Could you check a few things on this drawing? It's one solid part, dimensions in mm from its lowest x, y, z. Round coordinates to 2 decimals unless told otherwise and drop trailing zeros. Loops run counter-clockwise (first coordinate to the right, second up) from the corner with the lowest first, then second, coordinate; pieces in that order, holes last. Notation, with made-up numbers: M 62.25,6.25 L 102.25,6.25 A24 ccw 102.25,36.25 Z; hole C 33,-29 d9. An arc over 180 degrees is marked long. Return JSON: item names as keys, results as strings.
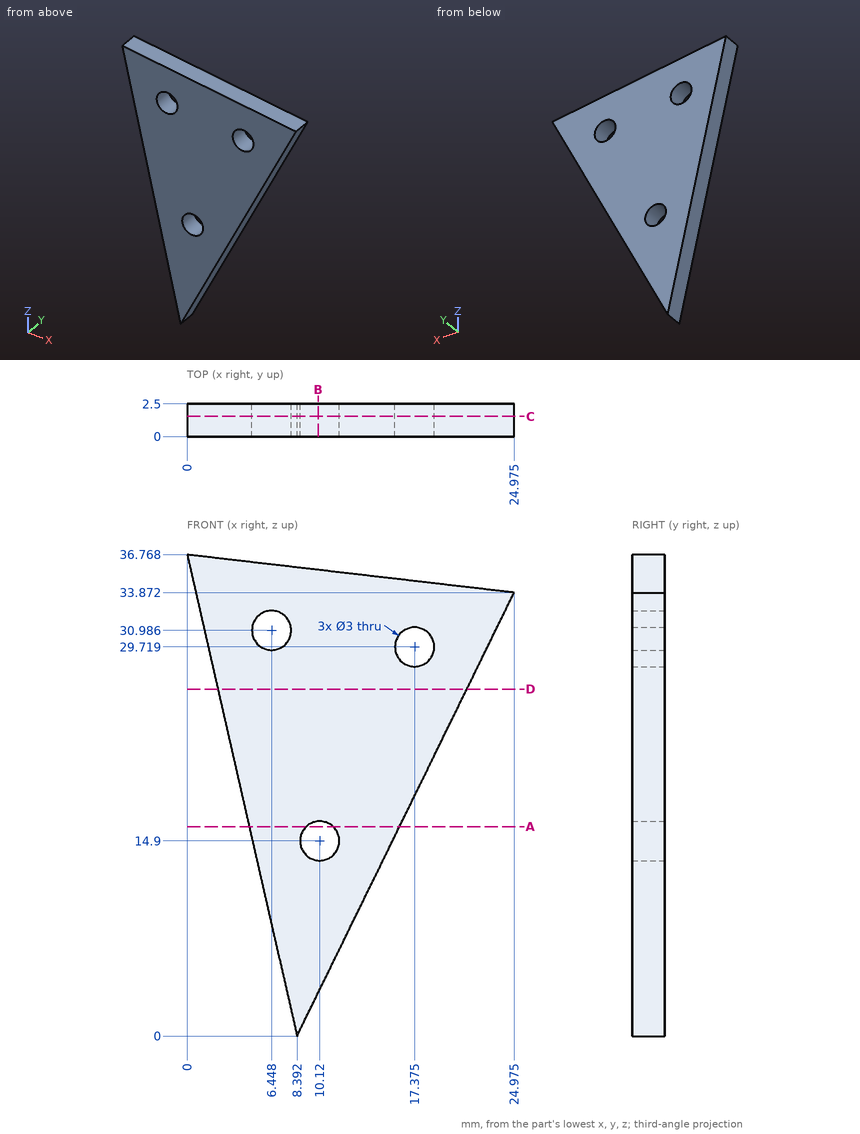
Q1. Suppose I cut it at B-B, the plane x = 10. Please give me the cut outline in (y, z) (1 decimal).
Results:
{"outline": "M 0,3.3 L 2.5,3.3 L 2.5,13.4 L 0,13.4 Z; M 0,16.4 L 2.5,16.4 L 2.5,35.6 L 0,35.6 Z"}
Q2. Suppose I cut it at C-C, the plane y = 1.55. Please give me the cut outline in (x, z) (1 decimal).
Results:
{"outline": "M 0,36.8 L 8.4,0 L 25,33.9 Z; hole C 6.4,31 d3; hole C 10.1,14.9 d3; hole C 17.4,29.7 d3"}
Q3. I'm going to push a flat-ended pin straight in: pin 1 Ø1.5 at (x, z) = (6, 10) entering from +Y. Where does the tip first touch, or does it pass through?
Results:
{"pin 1": "stops at y = 2.5"}
Q4. If I drill on line 1 along Z through (x, y) = (17.25, 0.35) (1 decimal); line 2 along Z through (x, y) = (18, 1.85) (1 decimal); line 3 along X through (y, z) = (2.35, 14.5) (1 decimal), over which ranges is the centre line in solid material (lowest first)?
Results:
{"line 1": "z = 18.1 to 28.2, 31.2 to 34.8", "line 2": "z = 19.6 to 28.4, 31.1 to 34.7", "line 3": "x = 5.1 to 8.7, 11.6 to 15.5"}
Q5. Suppose I cut it at A-A, the plane z = 16. Please give me the cut outline in (x, y) (1 decimal).
Results:
{"outline": "M 4.7,0 L 9.1,0 L 9.1,2.5 L 4.7,2.5 Z; M 11.1,0 L 16.2,0 L 16.2,2.5 L 11.1,2.5 Z"}
Q6. Suppose I cut it at D-D, the plane z = 26.5. Please give me the cut outline in (x, y) (1 decimal).
Results:
{"outline": "M 2.3,0 L 21.4,0 L 21.4,2.5 L 2.3,2.5 Z"}
